Read the model definition and answer for the solid it produces. Units are mm, in the model's axes. A direction names the side the tool comes from. Round coordinates to 2 decimals unless told otherwise and drop trailing zeros. Loops run counter-clockwise (first coordinate to the right, second up) from the corner with the lowest first, then second, coordinate; pieces in that order, holes last. Notation, with made-up numbers: (25.5, -31) -> (48.5, -31) arc R30 cw to (48.5, -8) -> close; hole circle Ø6 at (87.5, 2). An arc over 180 degrees is marked (long way). Put each result on its own line as item: value.
from build123d import *
from OCP.BRepFilletAPI import BRepFilletAPI_MakeChamfer

# Parameters (mm, degrees)
SKETCH1_W              = 16
SKETCH1_H              = 21
BOSS_EXTRUDE1_DEPTH    = 5.1
SKETCH2_R              = 1.85
CUT_EXTRUDE1_DEPTH     = 5.1
CHAMFER1_SIZE          = 3.1
CHAMFER1_SIZE2         = 0.830642497
SKETCH3_W              = 3.5
SKETCH3_H              = 1.5
BOSS_EXTRUDE2_DEPTH    = 10
CUT_EXTRUDE3_START     = -0.5
CUT_EXTRUDE3_OUTLINE_W = 13.8
CUT_EXTRUDE3_OUTLINE_H = 11.6
CUT_EXTRUDE3_DEPTH     = 0.5


# Read off the part's stored shape, not the designer's step: Cut-Extrude3
with BuildPart() as part:
    # Sketch1 → Boss-Extrude1 (new body)
    with BuildSketch(Plane(origin=(0, 0, 0), x_dir=(1, 0, 0), z_dir=(0, 1, 0))):
        with Locations((8, 10.5)):
            Rectangle(SKETCH1_W, SKETCH1_H)
    extrude(amount=BOSS_EXTRUDE1_DEPTH)

    # Sketch2 → Cut-Extrude1 (cut)
    with BuildSketch(Plane(origin=(0, 5.1, 0), x_dir=(1, 0, 0), z_dir=(0, 1, 0))):
        with Locations(Location((8, 15.3, 0), (0, 0, 270))):
            Circle(SKETCH2_R)
    extrude(amount=-CUT_EXTRUDE1_DEPTH, mode=Mode.SUBTRACT)

    # Chamfer1: one chamfer whose edges measure the first distance from different faces: ONE call of the kernel's chamfer builder (chamfer() names one face for all edges)
    chamfer1_edges_1 = [part.edges().sort_by_distance(p)[0] for p in [
        (16, 5.1, -10.5),
    ]]
    chamfer1_side_1 = [part.faces().sort_by_distance(p)[0] for p in [
        (16, 2.55, -10.5),
    ]]
    chamfer1_edges_2 = [part.edges().sort_by_distance(p)[0] for p in [
        (8, 5.1, -21),
    ]]
    chamfer1_side_2 = [part.faces().sort_by_distance(p)[0] for p in [
        (8, 2.55, -21),
    ]]
    chamfer1_edges_3 = [part.edges().sort_by_distance(p)[0] for p in [
        (0, 5.1, -10.5),
    ]]
    chamfer1_side_3 = [part.faces().sort_by_distance(p)[0] for p in [
        (0, 2.55, -10.5),
    ]]
    chamfer1_edges_4 = [part.edges().sort_by_distance(p)[0] for p in [
        (8, 5.1, 0),
    ]]
    chamfer1_side_4 = [part.faces().sort_by_distance(p)[0] for p in [
        (8, 2.55, 0),
    ]]
    chamfer1 = BRepFilletAPI_MakeChamfer(part.part.solid().wrapped)
    for e in chamfer1_edges_1:
        chamfer1.Add(CHAMFER1_SIZE, CHAMFER1_SIZE2, e.wrapped, chamfer1_side_1[0].wrapped)  # the first distance lies on this face
    for e in chamfer1_edges_2:
        chamfer1.Add(CHAMFER1_SIZE, CHAMFER1_SIZE2, e.wrapped, chamfer1_side_2[0].wrapped)  # the first distance lies on this face
    for e in chamfer1_edges_3:
        chamfer1.Add(CHAMFER1_SIZE, CHAMFER1_SIZE2, e.wrapped, chamfer1_side_3[0].wrapped)  # the first distance lies on this face
    for e in chamfer1_edges_4:
        chamfer1.Add(CHAMFER1_SIZE, CHAMFER1_SIZE2, e.wrapped, chamfer1_side_4[0].wrapped)  # the first distance lies on this face
    add(Compound.cast(chamfer1.Shape()), mode=Mode.REPLACE)

    # Sketch3 → Boss-Extrude2 (add)
    with BuildSketch(Plane.XY):
        with Locations((2.75, 1.05)):
            Rectangle(SKETCH3_W, SKETCH3_H)
        with Locations((13.25, 1.05)):
            Rectangle(SKETCH3_W, SKETCH3_H)
    extrude(amount=BOSS_EXTRUDE2_DEPTH)

    # Cut-Extrude3 outline → Cut-Extrude3 (cut)
    with BuildSketch(Plane(origin=(0, 0, 0), x_dir=(-1, 0, 0), z_dir=(0, -1, 0)).offset(CUT_EXTRUDE3_START)):
        with Locations((-8, 6.8)):
            Rectangle(CUT_EXTRUDE3_OUTLINE_W, CUT_EXTRUDE3_OUTLINE_H)
    extrude(amount=CUT_EXTRUDE3_DEPTH, mode=Mode.SUBTRACT)


solid = part.part
Item 1: The part is cut by section A-A (z = -15.3). Determine the outline of the cut face in (x, y), then the cut area to 3 significant figures.
Derived:
outline: (0, 0) -> (6.15, 0) -> (6.15, 5.1) -> (0.83, 5.1) -> (0, 2) -> close; (9.85, 0) -> (16, 0) -> (16, 2) -> (15.17, 5.1) -> (9.85, 5.1) -> close
area: 60.2 mm^2
Item 2: The part is cut by section D-D (z = -8.5). Determine the outline of the cut face in (x, y), then the cut area to 3 significant figures.
Derived:
outline: (0, 0) -> (1.1, 0) -> (1.1, 0.5) -> (14.9, 0.5) -> (14.9, 0) -> (16, 0) -> (16, 2) -> (15.17, 5.1) -> (0.83, 5.1) -> (0, 2) -> close
area: 72.1 mm^2
Item 3: The part is cut by section B-B (x = 8). Determine the outline of the cut face in (y, z), then the cut area to 3 significant figures.
Derived:
outline: (0, -21) -> (2, -21) -> (5.1, -20.17) -> (5.1, -17.15) -> (0, -17.15) -> close; (0, -13.45) -> (5.1, -13.45) -> (5.1, -0.83) -> (2, 0) -> (0, 0) -> (0, -1) -> (0.5, -1) -> (0.5, -12.6) -> (0, -12.6) -> close
area: 79.9 mm^2
Item 4: For a pull along Z with two mould halves and no side action, classify faces 1 (the flat face through (8, 0.5, -7)), 2 (the cylindrical face through (8.08, 2.59, -17.15)), 3 (the flat face through (11.5, 1, 5)), 4 (the flat face through (7.89, 3.57, -0.42)) as pulls with the +Z half, pulls with the -Z half, needs draft (parallel to the pull), parting line crosses it, or undercut.
Derived:
face 1: undercut
face 2: undercut
face 3: needs draft
face 4: pulls with the +Z half
Item 5: Which of the six approach directions +Z, -Z, +X, -X, +Y, -Y give full straight-line access (tool end or side, diameter ignored) to faces 5 (the flat face through (1, 1, 5)), 6 (the flat face through (4.5, 1, 5)), 7 (the flat face through (13, 1.8, 5))?
Derived:
face 5: +Z, -X, +Y, -Y
face 6: +Z, +Y, -Y
face 7: +Z, +X, -X, +Y
Item 6: The part is cut by section C-C (y = 1.5). Determine the outline of the cut face in (x, z).
Derived:
outline: (0, -21) -> (16, -21) -> (16, 0) -> (15, 0) -> (15, 10) -> (11.5, 10) -> (11.5, 0) -> (4.5, 0) -> (4.5, 10) -> (1, 10) -> (1, 0) -> (0, 0) -> close; hole circle Ø3.7 at (8, -15.3)
Item 7: Flat-ended cylindrical pins translate along their axes: pin 1 Ø4 at (x, z) = (2, 4) entering from -Y; pin 2 Ø1.2 at (y, z) = (1, 7) entering from +X; pin 3 Ø1 at (x, z) = (12.5, 7) entering from +Y. Find the tip coordinate at first contact, or state that the pin passes through.
Derived:
pin 1: stops at y = 0.3
pin 2: stops at x = 15
pin 3: stops at y = 1.8
Item 8: Find the intervals of material crossed by line 1 along X through (y, z) = (1.1, -15.3); line 2 along X through (y, z) = (0.4, -11); line 3 along Y through (x, z) = (14, 2), in increasing order.
Derived:
line 1: x = 0 to 6.15, 9.85 to 16
line 2: x = 0 to 1.1, 14.9 to 16
line 3: y = 0.3 to 1.8
